Geometry: final body of the model. Coordinates: model frame, mm. Face numbers are marked on the shaded views. A direction names the side the tool comes from. Give positions to 0.01 mm unless a question says otherwise; leave off trailing zeros. Write each loop counter-clockwise with the first axis right and the second up, starting at its lowest first coordinate (ties: lowest second). Pieces come first, ordered by that corner, then holes.
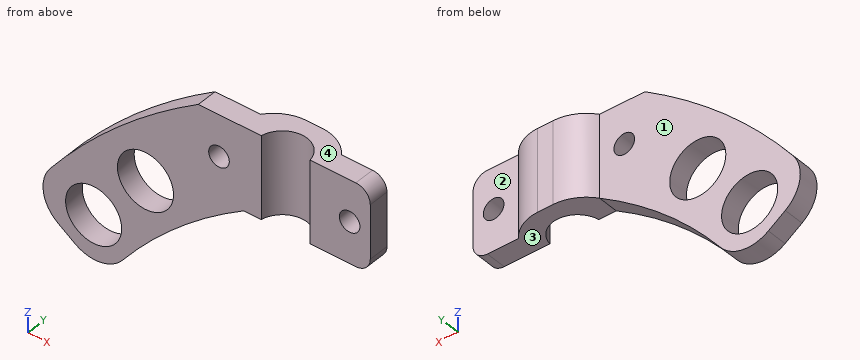
Autodesk Fusion 360 part; units mm, degrees
sketch "Sketch1" plane through (0, 0, 0) normal (0, 0, 1) x (1, 0, 0)
  line L0 (0, 0) -> (15, 0) construction
  arc A0 (8.9159, -9.9997) -> (9.0729, 9.9997) centre (8.9986, 0) ccw
  line L1 (9.0729, 9.9997) -> (5.3447, 10.0008)
  arc A1 (5.3447, 10.0008) -> (5.3451, -10.0008) centre (5.3418, 0) ccw
  line L2 (5.3451, -10.0008) -> (8.9159, -9.9997)
  line L3 (0.0839, 1) -> (-13.6592, 1)
  line L4 (-13.6592, 1) -> (-13.6592, 6)
  line L5 (-13.6592, 6) -> (-2.6592, 6)
  line L6 (0.0839, 1) -> (27.9986, 1)
  line L7 (27.9986, 1) -> (27.9986, 6)
  line L8 (27.9986, 6) -> (16.9986, 6)
  circle A2 centre (7.5, 0) radius 6
  dimension "d4" = 5
  dimension "d6" = 5
  dimension "d7" = 1
  dimension "d8" = 1
  dimension "d52" = 11
  dimension "d53" = 11
  dimension "d122" = 12
extrude "Extrude1" add sketch "Sketch1" along normal blind 20 contours A0 L1 A1 L3 L6 A2 | A0 L6 L7 L8 | A1 L3 L4 L5
hole "Hole1" at (-8.6592, 6, 10) direction (0, -1, 0) diameter 5 depth 5 tip angle 118
hole "Hole2" at (22.9986, 6, 10) direction (0, -1, 0) diameter 5 depth 5 tip angle 118
fillet "Fillet9" radius 3.5 2 edges at (27.9986, 3.5, 20) (27.9986, 3.5, 0)
sketch "Sketch7" plane through (0, 6, 0) normal (0, 1, 0) x (-1, 0, 0)
  circle A0 centre (8.6592, 10) radius 2.5
  line L0 (2.6592, 0) -> (13.6592, 0)
  line L1 (13.6592, 0) -> (13.6592, 20)
  line L2 (13.6592, 20) -> (2.6592, 20)
  line L3 (2.6592, 20) -> (2.6592, 0)
  line L4 (36.6932, -32.7022) -> (54.7147, -20.0838)
  line L5 (13.6592, 0) -> (2.6592, 0)
  circle A1 centre (39.0344, -18.8185) radius 6.8
  circle A2 centre (26.4668, -4.5455) radius 6.8
  line L6 (45.7039, -26.393) -> (13.6592, 10) construction
  circle A3 centre (39.0344, -18.8185) radius 8.75 construction
  circle A4 centre (26.4668, -4.5455) radius 8.75 construction
  arc A5 (54.7147, -20.0838) -> (13.6592, 20) centre (-60.9979, -97.5341) ccw
  arc A6 (36.6932, -32.7022) -> (2.6592, 0) centre (-53.2733, -92.2713) ccw
  dimension "d109" = 22
  dimension "d111" = 40
  dimension "d112" = 13.6
  dimension "d113" = 13.6
  dimension "d114" = 17.5
  dimension "d115" = 17.5
extrude "Extrude9" add sketch "Sketch7" against normal blind 5 contours L0 L1 L4 L5 A5 A6
fillet "Fillet8" radius 8.5 2 edges at (-54.7147, 3.5, -20.0838) (-36.6932, 3.5, -32.7022)
equation "d6 = d4"
equation "d8 = d7"
Q1. Section C-C on z = -2.5. Output: boundary loops of the cut face in (x, y), plus the area to 3 significant figures.
Filled sheet:
outline: (-40.77, 1) - (-32.95, 1) - (-32.95, 6) - (-40.77, 6) - close; (-19.98, 1) - (-6.59, 1) - (-6.59, 6) - (-19.98, 6) - close
area: 106 mm2
Q2. Access query for the marked faces 1, 2, 3 and 4. Directions: +Z, -Z, +X, -X, +Y, -Y. A direction counts if a zero-diameter tool reaches every point of the face in a straight line with its end or side. Return the directions, or none.
Filled sheet:
face 1: +Z, -Z, -X, +Y
face 2: +Z, -Z, +X, +Y
face 3: -Z, +X, +Y, -Y
face 4: +Z, +X, -X, +Y, -Y
Q3. Section D-D on x = 7. Output: boundary loops of the cut face in (y, z).
Filled sheet:
outline: (5.98, 0) - (10, 0) - (10, 20) - (5.98, 20) - close
Q4. Pin query (flat end, axial travel): P1, Ø8, axis at x = -26.47, z = -4.55, coming from the -Y side; P2, Ø8, axis at x = -19.5, z = -13.5, coming from the +Y side; P3, Ø3, axis at y = 4.5, z = 11.5, coming from the -X side; P4, Ø5, axis at y = 5.5, z = -4, coming from the +X side. Return the tip coordinate at first contact, or that it passes through.
Filled sheet:
P1: passes through
P2: stops at y = 6
P3: stops at x = -27.46
P4: stops at x = -5.06
Q5. Section A-A on y = 2.5. Output: boundary loops of the cut face in (x, z), plus the area to 3 significant figures.
Filled sheet:
outline: (-49.55, -12.88) arc R8.5 ccw to (-47.68, -25.01) - (-43.57, -27.89) arc R8.5 ccw to (-31.98, -26.13) arc R107.9 cw to (-2.66, 0) - (2.05, 0) - (2.05, 20) - (-13.66, 20) arc R139.24 ccw to start; (12.95, 0) - (24.5, 0) arc R3.5 ccw to (28, 3.5) - (28, 16.5) arc R3.5 ccw to (24.5, 20) - (12.95, 20) - close; hole circle Ø13.6 at (-39.03, -18.82); hole circle Ø13.6 at (-26.47, -4.55); hole circle Ø5 at (-8.66, 10); hole circle Ø5 at (23, 10)
area: 1,310 mm2
Q6. Section B-B on z = 10. Output: boundary loops of the cut face in (x, y).
Filled sheet:
outline: (-27.46, 1) - (-11.16, 1) - (-11.16, 6) - (-27.46, 6) - close; (-6.16, 1) - (1.58, 1) arc R6 cw to (13.42, 1) - (20.5, 1) - (20.5, 6) - (17, 6) arc R10 ccw to (9.07, 10) - (5.34, 10) arc R10 ccw to (-2.66, 6) - (-6.16, 6) - close; (25.5, 1) - (28, 1) - (28, 6) - (25.5, 6) - close
Q7. Ray query, line 1 along X through (y, z) = (3.35, 10); line 2 along X through (y, z) = (3, 10); line 3 along Z through (x, y) = (19, 4.25). Return the intervals inside material, ascending.
Filled sheet:
line 1: x = -27.46 to -11.16, -6.16 to 2.52, 12.48 to 20.5, 25.5 to 28
line 2: x = -27.46 to -11.16, -6.16 to 2.3, 12.7 to 20.5, 25.5 to 28
line 3: z = 0 to 20
